Verification items for the finished model (mm, model axes). Face numbers are marked on the shaded views. Coordinates: 2 decimals unless noted, no trailing zeros. Order: outer loops, then holes, each group sorted by start corner. A loop starts at its lowest first (then second) coordinate and runs counter-clockwise, first axis right, second up. Notation, with made-up numbers: M 16,27.5 L 21,27.5 A11 ccw 21,38.5 Z; hole C 60.5,34 d5. An arc over 180 degrees is marked long. Write item = value, one per line.
Autodesk Inventor part; units mm, degrees
ref_plane "YZ Plane" through (0, 0, 0) normal (1, 0, 0) x (0, 1, 0)
ref_plane "XZ Plane" through (0, 0, 0) normal (0, 1, 0) x (-1, 0, 0)
ref_plane "XY Plane" through (0, 0, 0) normal (0, 0, 1) x (1, 0, 0)
sketch "Boceto1" plane through (0, 0, 0) normal (0, 1, 0) x (-1, 0, 0)
  circle A0 centre (0, 0) radius 75
  circle A1 centre (0, 0) radius 40
  dimension "d0" = 150
  dimension "d1" = 80
extrude "Extrusión1" add sketch "Boceto1" along normal blind 25
sketch "Boceto2" plane through (0, 0, 0) normal (0, -1, 0) x (1, 0, 0)
  circle A0 centre (0, 0) radius 47
  dimension "d4" = 94
extrude "Extrusión2" cut sketch "Boceto2" against normal blind 16
sketch "Boceto3" plane through (0, 25, 0) normal (0, 1, 0) x (1, 0, 0)
  circle A0 centre (0, 0) radius 61
  line L0 (0, 0) -> (61, 0) construction
  point P0 (30.5, 52.8275)
  point P1 (-30.5, 52.8275)
  point P2 (-61, 0)
  point P3 (-30.5, -52.8275)
  point P4 (30.5, -52.8275)
  dimension "d7" = 122
  dimension "d10" = 360
hole "Agujero1" at (61, 25, 0) at (30.5, 25, -52.8275) at (-30.5, 25, -52.8275) at (-61, 25, 0) at (-30.5, 25, 52.8275) at (30.5, 25, 52.8275) direction (0, -1, 0) diameter 10.106 depth 1.75
properties part number "9_AnilloComplementarioA"
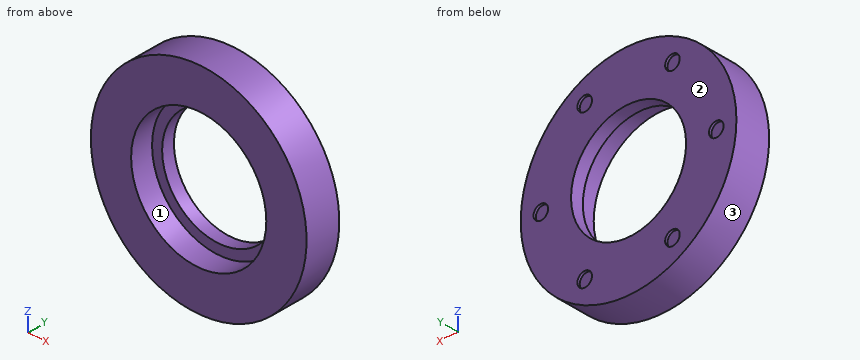
Item 1: Scan lines: L1, parallel to Z at x = 0, y = 4; L2, parallel to Z at x = 0, y = 22.5; L3, parallel to Z at x = 30.5, y = 24.25. Record each from-to range of solid material in increasing order. Write a range as from..to.
Report:
L1 = -75..-47, 47..75
L2 = -75..-40, 40..75
L3 = -68.52..-57.88, -47.77..-25.88, 25.88..47.77, 57.88..68.52
Item 2: Sectioned sample at B-B, the plane z = 14. Enter the section's corners in (x, y).
Report:
outline = M -73.68,0 L -44.87,0 L -44.87,16 L -37.47,16 L -37.47,25 L -73.68,25 Z; M 37.47,16 L 44.87,16 L 44.87,0 L 73.68,0 L 73.68,25 L 37.47,25 Z
Item 3: Release check for a two-part mould opening along X. For the marked faces 1, 2 and 3 record: pulls with the +X half, pulls with the -X half, needs draft (parallel to the pull), parting line crosses it, or undercut.
Report:
face_1 = undercut
face_2 = needs draft
face_3 = parting line crosses it
Item 4: Gauge pin test, flat ends, axial feed: pin 1 (12 mm diameter, centred on x = 31, y = 11.5, fed in from +Z); pin 2 (3 mm diameter, centred on x = 30, z = 55.5, fed in from +Y); pin 3 (5 mm diameter, centred on x = 46.5, y = 16, fed in from -Z); pin 4 (2 mm diameter, centred on x = 60, z = 49, fed in from +Y). Record the tip position at first contact, or that the pin passes through.
Report:
pin_1 = 70.71
pin_2 = 23.25
pin_3 = -60.74
pin_4 = through
Item 5: Sectioned sample at D-D, the plane y = 5. Enter the section's corners in (x, z), then the cut area to 3 significant figures.
Report:
outline = C 0,0 d150; hole C 0,0 d94
area = 10,700 mm^2
Item 6: Sectioned sample at C-C, the plane x = -63. Enter the section's corners in (y, z), then the cut area to 3 significant figures.
Report:
outline = M 0,-40.69 L 25,-40.69 L 25,-4.64 L 23.25,-4.64 L 23.25,4.64 L 25,4.64 L 25,40.69 L 0,40.69 Z
area = 2,020 mm^2
Item 7: Sectioned sample at A-A, the plane x = 0. Enter the section's corners in (y, z).
Report:
outline = M 0,-75 L 25,-75 L 25,-40 L 16,-40 L 16,-47 L 0,-47 Z; M 0,47 L 16,47 L 16,40 L 25,40 L 25,75 L 0,75 Z
